from build123d import *

# Parameters (mm, degrees)
F1_DEPTH    = 2
F0_W        = 6
F0_H        = 5.0999999046
F2_DEPTH    = 1.1
F3_W        = 2.7999999523
F3_H        = 0.2000000477
F4_DEPTH    = 2.0463333095
F5_R        = 1.2711666667
F6_DEPTH    = 8.5
F7_R        = 0.5833333333
F8_DEPTH    = 3
F9_R        = 0.8728333333
F10_DEPTH   = 7.7
F11_SIZE2   = 0.692820323
F11_SIZE    = 1.2
F11_2_SIZE2 = 0.692820323
F11_2_SIZE  = 1.2
F13_DEPTH   = 12.5
F14_SCALE   = 3


with BuildPart() as f1:
    # F0 (on Front) → F1 (new body, symmetric)
    with BuildSketch(Plane.XZ):
        Polygon((-6, 5.0999999046), (0, 5.0999999046), (2.5, 5.0999999046), (2.5, 9.6999998093), (-0.9000000954, 9.6999998093), (-0.9000000954, 13.6999998093), (-1.6000000834, 13.6999998093), (-1.6000000834, 9.8999998569), (-2.2463334168, 9.8999998569), (-2.2463334168, 13.6999998093), (-2.9463334049, 13.6999998093), (-2.9463334049, 9.6999998093), (-6, 9.6999998093), align=None)
    extrude(amount=F1_DEPTH, both=True)

    # F0 (on Front) → F2 (join, symmetric)
    with BuildSketch(Plane.XZ):
        with Locations((-3, 2.5499999523)):
            Rectangle(F0_W, F0_H)
    extrude(amount=F2_DEPTH, both=True)

    # F3 (on face) → F4 (cut, through all)
    with BuildSketch(Plane.YZ.offset(-0.9000000954)):
        with Locations((0, 13.7999998331)):
            Rectangle(F3_W, F3_H)
        with BuildLine():
            Line((-1.3999999762, 13.6999998093), (-1.3999999762, 12.4999998808))
            ThreePointArc((-1.3999999762, 12.4999998808), (0, 11.0999999046), (1.3999999762, 12.4999998808))
            Line((1.3999999762, 12.4999998808), (1.3999999762, 13.6999998093))
            Line((1.3999999762, 13.6999998093), (-1.3999999762, 13.6999998093))
        make_face()
    extrude(amount=-F4_DEPTH, mode=Mode.SUBTRACT)

    # F5 (on face) → F6 (cut)
    with BuildSketch(Plane.YZ.offset(2.5)):
        with Locations((0, 6.6999998093)):
            Circle(F5_R)
    extrude(amount=-F6_DEPTH, mode=Mode.SUBTRACT)

    # F7 (on face) → F8 (cut)
    with BuildSketch(Plane.XY.offset(9.6999998093)):
        with Locations((0.3999998569, 0)):
            Circle(F7_R)
    extrude(amount=-F8_DEPTH, mode=Mode.SUBTRACT)

    # F9 (on face) → F10 (cut)
    with BuildSketch(Plane.XY.offset(9.6999998093)):
        with Locations((-4.6463334525, 0)):
            Circle(F9_R)
    extrude(amount=-F10_DEPTH, mode=Mode.SUBTRACT)

    # F11
    f11_edges = [f1.edges().sort_by_distance(p)[0] for p in [
        (-3, -1.1, 0),
    ]]
    f11_side = f1.faces().sort_by_distance((-3, -1.1, 2.55))[0]
    chamfer(f11_edges, length=F11_SIZE, length2=F11_SIZE2, reference=f11_side)

    # F11#2
    f11_2_edges = [f1.edges().sort_by_distance(p)[0] for p in [
        (-3, 1.1, 0),
    ]]
    f11_2_side = f1.faces().sort_by_distance((-3, 1.1, 2.55))[0]
    chamfer(f11_2_edges, length=F11_2_SIZE, length2=F11_2_SIZE2, reference=f11_2_side)

    # F12 (on Front) → F13 (cut, symmetric)
    with BuildSketch(Plane.XZ):
        Polygon((-2.5119182901, 0.0119182901), (-3, 0.5), (-3.4880817099, 0.0119182901), (-4.0324307496, 0.5562673297), (-4.4787575401, 0.1099405392), (-5.1049532346, 0.7361362337), (-5.518700193, 0.3223892754), (-6, 0.8036890823), (-6, 0), (0, 0), (0, 0.8036890823), (-0.481299807, 0.3223892754), (-0.8950467654, 0.7361362337), (-1.5212424599, 0.1099405392), (-1.9675692504, 0.5562673297), align=None)
    extrude(amount=F13_DEPTH, both=True, mode=Mode.SUBTRACT)


with BuildPart() as f1_1:
    # F14: moved
    add(f1.part.scale(F14_SCALE))


solid = f1_1.part
Check sheet for the modelled part. Datum: model origin and axes. Units: mm. A direction names the side the tool comes from. Coordinates: 2 decimals unless noted, no trailing zeros. Loops run counter-clockwise (first coordinate to the right, second up) from the corner with the lowest first, then second, coordinate; pieces in that order, holes last. Notation, with made-up numbers: (49, 33) -> (54, 33) arc R28 cw to (54, 62) -> close; hole circle Ø8 at (47.5, -12). An arc over 180 degrees is marked (long way). Answer in a Markdown table with one row per item.
1. Material ranges on line 1 along X through (y, z) = (0, 25); line 2 along X through (y, z) = (0, 11.75); line 3 along Z through (x, y) = (6.25, 0), recorded low to high. Write a range as [from, to].
Check values:
| item | result |
|---|---|
| line 1 | x = [-18, -16.56], [-11.32, -0.55], [2.95, 7.5] |
| line 2 | x = [-18, -16.56], [-11.32, 0] |
| line 3 | z = [15.3, 16.29], [23.91, 29.1] |
2. Sectioned sample at A-A, the plane z = 20.1. Record the boundary of the cut face in (x, y).
Check values:
| item | result |
|---|---|
| outline | (-18, -6) -> (7.5, -6) -> (7.5, -3.81) -> (-18, -3.81) -> close; (-18, 3.81) -> (7.5, 3.81) -> (7.5, 6) -> (-18, 6) -> close |
3. Release check for a two-part mould opening along X. For faces 5 (the face through (-12.757, -0.031, 1.009)), 6 (the face through (-8.839, 0, 33)), 7 (the face through (-3.7, -0.1, 33.3)) record: released by +X, released by -X, zero draft, split by the parting line, or undercut.
Check values:
| item | result |
|---|---|
| face 5 | undercut |
| face 6 | released by -X |
| face 7 | zero draft |
4. Sectioned sample at D-D, the plane x = -2. Record the boundary of the cut face in (y, z), then the cut area to 3 significant figures.
Check values:
| item | result |
|---|---|
| outline | (-6, 15.3) -> (-3.3, 15.3) -> (-3.3, 3.6) -> (-2.1, 1.52) -> (2.1, 1.52) -> (3.3, 3.6) -> (3.3, 15.3) -> (6, 15.3) -> (6, 29.1) -> (-6, 29.1) -> close; hole circle Ø7.63 at (0, 20.1) |
| area | 208 mm2 |
5. Sectioned sample at C-C, the plane y = 0. Give the number of separate pieces and of enclosed holes in the cut face, then the cut area to 3 significant figures.
Check values:
| item | result |
|---|---|
| separate pieces | 4 |
| enclosed holes | 0 |
| area | 331 mm2 |
6. Go/stop test with flat-tipped pins: pin 1 (1.6 mm diameter, centred on x = -6, y = -0.5, fed in from +Z); pin 2 (5 mm diameter, centred on x = -8.5, y = 0.5, fed in from +Z); pin 3 (4 mm diameter, centred on x = -11, y = 4.5, fed in from +Z). Record where each tip stops, or that it passes through.
Check values:
| item | result |
|---|---|
| pin 1 | stops at z = 33.38 |
| pin 2 | stops at z = 34.56 |
| pin 3 | stops at z = 29.1 |
7. Access from +Z, -Z, +X, -X, +Y, -Y to the whole of each face (thin tool, end or side, straight path). Record for faces 1 (the face through (-4, -4.2, 39)), 2 (the face through (-6, 0, 29.7)), 3 (the face through (-9, -3.3, 10)), 4 (the face through (-2.056, -0.035, 1.579)).
Check values:
| item | result |
|---|---|
| face 1 | +Z, +X, -X |
| face 2 | +Z, +Y, -Y |
| face 3 | -Z, +X, -X, -Y |
| face 4 | -Z, +Y, -Y |
8. Sectioned sample at B-B, the plane x = 3.5. Record the boundary of the cut face in (y, z), then the cut area to 3 significant figures.
Check values:
| item | result |
|---|---|
| outline | (-6, 15.3) -> (6, 15.3) -> (6, 29.1) -> (-6, 29.1) -> close; hole circle Ø7.63 at (0, 20.1) |
| area | 120 mm2 |
